The model under review builds one solid part; all positions refer to its coordinate system, in mm. Face numbers are marked on the shaded views. A direction names the side the tool comes from. Round coordinates to 2 decimals unless told otherwise and drop trailing zeros. Write each loop counter-clockwise with the first axis right and the second up, starting at its lowest first coordinate (ties: lowest second). Pieces come first, ordered by that corner, then holes.
Item 1: To check wall thickness, follow L1, parallel to Y at x = 24, z = -3; L2, parallel to Z at x = -3, y = -22; L3, parallel to Z at x = -9.5, y = -17.5. State the ranges of each line that lie inside material, in increasing order.
Item 2: Add section B-B (z = 0). Give the boundary of the cut face in (x, y).
Item 3: Add section D-D (x = 9). Give the boundary of the cut face in (y, z), plus the area to 3 significant figures.
Item 4: Add section A-A (y = -7.5). Give the boundary of the cut face in (x, z), plus the area to 3 significant figures.
Item 5: Machinability: for the marked faces 1 and 2, which of the approach directions +Z, -Z, +X, -X, +Y, -Y give a long, thin tool a straight path to every point of the face, cutting with its end or side? Answer none if there is none.
Item 6: Add section C-C (z = -7). Give the boundary of the cut face in (x, y), plus the area to 3 significant figures.
Item 7: Clearance check with flat-ended pins moving along their axes: pin 1 Ø10 at (x, y) = (19, -20) entering from +Z; pin 2 Ø4 at (x, z) = (-21.5, -4.5) entering from -Y; pin 3 Ø5.5 at (x, z) = (20.62, 11.91) entering from +Y. State where each tip first meets the part, or that it passes through.
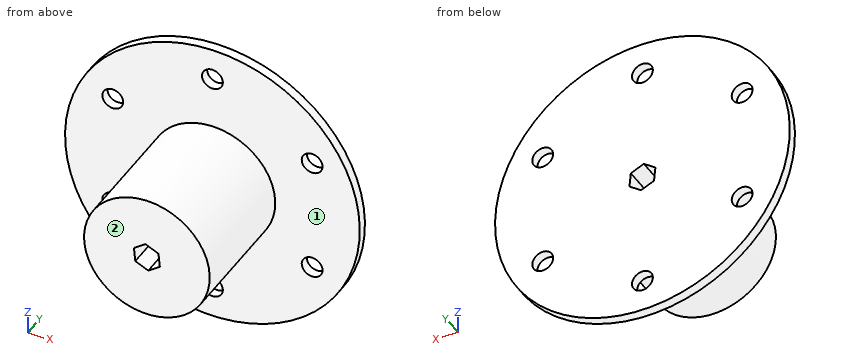
```python
from build123d import *

# Parameters (mm, degrees)
SKETCH1_R           = 30.48
SKETCH1_R_2         = 2.15265
BOSS_EXTRUDE1_DEPTH = 2
CUT_EXTRUDE1_DEPTH  = 10
SKETCH3_R           = 13
BOSS_EXTRUDE2_DEPTH = 25.4


with BuildPart() as part:
    # Sketch1 → Boss-Extrude1 (new body)
    with BuildSketch(Plane(origin=(0, 0, 0), x_dir=(1, 0, 0), z_dir=(0, 1, 0))):
        with Locations(Location((0, 0, 0), (0, 0, 270))):
            Circle(SKETCH1_R)
        with Locations(Location((0, -23.8125, 0), (0, 0, 270))):
            Circle(SKETCH1_R_2, mode=Mode.SUBTRACT)
        with Locations(Location((20.622229928, -11.90625, 0), (0, 0, 270))):
            Circle(SKETCH1_R_2, mode=Mode.SUBTRACT)
        with Locations(Location((20.622229928, 11.90625, 0), (0, 0, 270))):
            Circle(SKETCH1_R_2, mode=Mode.SUBTRACT)
        with Locations(Location((0, 23.8125, 0), (0, 0, 270))):
            Circle(SKETCH1_R_2, mode=Mode.SUBTRACT)
        with Locations(Location((-20.622229928, 11.90625, 0), (0, 0, 270))):
            Circle(SKETCH1_R_2, mode=Mode.SUBTRACT)
        with Locations(Location((-20.622229928, -11.90625, 0), (0, 0, 270))):
            Circle(SKETCH1_R_2, mode=Mode.SUBTRACT)
    extrude(amount=BOSS_EXTRUDE1_DEPTH)

    # Sketch2 → Cut-Extrude1 (cut)
    with BuildSketch(Plane(origin=(0, 2, 0), x_dir=(1, 0, 0), z_dir=(0, 1, 0))):
        Polygon((-2.680603767, -1.218344551), (-0.285184552, -2.930643235), (2.395419215, -1.712298684), (2.680603767, 1.218344551), (0.285184552, 2.930643235), (-2.395419215, 1.712298684), align=None)
    extrude(amount=-CUT_EXTRUDE1_DEPTH, mode=Mode.SUBTRACT)

    # Sketch3 → Boss-Extrude2 (add)
    with BuildSketch(Plane.XZ):
        with Locations(Location((0, 0, 0), (0, 0, 90))):
            Circle(SKETCH3_R)
        Polygon((-0.285184552, 2.930643235), (-2.680603767, 1.218344551), (-2.395419215, -1.712298684), (0.285184552, -2.930643235), (2.680603767, -1.218344551), (2.395419215, 1.712298684), align=None, mode=Mode.SUBTRACT)
    extrude(amount=BOSS_EXTRUDE2_DEPTH)


solid = part.part
```
Numbers:
1. L1: y = 0 to 2
1. L2: z = -12.65 to 12.65
1. L3: z = -8.87 to 8.87
2. outline: (-30.48, 0) - (-13, 0) - (-13, -25.4) - (-2.56, -25.4) - (-2.56, 2) - (-30.48, 2) - close; (2.56, -25.4) - (13, -25.4) - (13, 0) - (30.48, 0) - (30.48, 2) - (2.56, 2) - close
3. outline: (-25.4, -9.38) - (0, -9.38) - (0, -29.12) - (2, -29.12) - (2, 29.12) - (0, 29.12) - (0, 9.38) - (-25.4, 9.38) - close
3. area: 593 mm2
4. outline: circle Ø26 at (0, 0); hole (-2.68, 1.22) - (-2.4, -1.71) - (0.29, -2.93) - (2.68, -1.22) - (2.4, 1.71) - (-0.29, 2.93) - close
4. area: 508 mm2
5. face 1: -Y
5. face 2: +Z, -Z, +X, -X, -Y
6. outline: (-29.67, 0) - (-10.95, 0) - (-10.95, -25.4) - (10.95, -25.4) - (10.95, 0) - (29.67, 0) - (29.67, 2) - (-29.67, 2) - close
6. area: 675 mm2
7. pin 1: passes through
7. pin 2: stops at y = 0
7. pin 3: stops at y = 2
